```python
from build123d import *

# Parameters (mm, degrees)
F0_W     = 520.7
F0_H     = 520.7
F0_R     = 203.2
F1_DEPTH = 19.05
F3_DEPTH = 10


with BuildPart() as f1:
    # F0 (on Top) → F1 (new body)
    with BuildSketch(Plane.XY):
        Rectangle(F0_W, F0_H)
        Circle(F0_R, mode=Mode.SUBTRACT)
    extrude(amount=F1_DEPTH)

    # F2 (on face) → F3 (join)
    with BuildSketch(Plane.XY.offset(19.05)):
        Polygon((98.70539, 125.646158), (125.646158, 98.70539), (188.507951, 161.567183), (161.567183, 188.507951), align=None)
    extrude(amount=F3_DEPTH)


solid = f1.part
```
The model under review builds one solid part; all positions refer to its coordinate system, in mm. A direction names the side the tool comes from. Round coordinates to 2 decimals unless told otherwise and drop trailing zeros. Order: outer loops, then holes, each group sorted by start corner. A loop starts at its lowest first (then second) coordinate and runs counter-clockwise, first axis right, second up. Notation, with made-up numbers: (20.5, 50) -> (71.5, 50) arc R12 cw to (71.5, 60) -> close; hole circle Ø8 at (-38.75, -13). An arc over 180 degrees is marked (long way). One line per item, written item: value. Start each with the question number.
Q1. Clearance check with a flat-ended pin moving along its axis: pin 1 Ø1 at (x, y) = (196.5, -197) entering from +Z. State where the tip first meets the part, or that it passes through.
Q2. Machinability: for faces 5 (the face through (156.64, 129.7, 23.98)), 6 (the face through (175.226, 174.849, 23.98)), 7 (the face through (-4, -260.35, 9)), which of the approach directions +Z, -Z, +X, -X, +Y, -Y give a long, thin tool a straight path to every point of the face, cutting with its end or side? Answer none if there is none.
Q3. Take a section at A-A (x = 0). Write out the cut boundary in (y, z).
Q4. Take a section at C-C (z = 6). Write out the cut boundary in (x, y).
Q5. Wall thickness on line 1 (Y direction, x = 0, z = 5); line 2 (Y direction, x = -4.5, z = 1.75): over which ranges is each line inside the solid? List them lowest first.
Q6. Mouldability with a two-part tool opening along X and no side actions: class faces 1 (the face through (260.35, -4, 9)), 2 (the face through (-177, -112, 19.05)), 3 (the face through (127, 128, 19.05)), 4 (the face through (130.58, 157.52, 23.98)) as released by +X, released by -X, zero draft, split by the parting line, or undercut.
Q7. Take a section at D-D (x = 225). Write out the cut boundary in (y, z), and give its area (3 significant figures).
Reported:
1. pin 1: stops at z = 19.05
2. face 5: +Z, +X, -Y
2. face 6: +Z, +X, +Y
2. face 7: +Z, -Z, +X, -X, -Y
3. outline: (-260.35, 0) -> (-203.2, 0) -> (-203.2, 19.05) -> (-260.35, 19.05) -> close; (203.2, 0) -> (260.35, 0) -> (260.35, 19.05) -> (203.2, 19.05) -> close
4. outline: (-260.35, -260.35) -> (260.35, -260.35) -> (260.35, 260.35) -> (-260.35, 260.35) -> close; hole circle Ø406.4 at (0, 0)
5. line 1: y = -260.35 to -203.2, 203.2 to 260.35
5. line 2: y = -260.35 to -203.15, 203.15 to 260.35
6. face 1: released by +X
6. face 2: zero draft
6. face 3: undercut
6. face 4: released by -X
7. outline: (-260.35, 0) -> (260.35, 0) -> (260.35, 19.05) -> (-260.35, 19.05) -> close
7. area: 9,920 mm2
